Check sheet for the modelled part. Datum: model origin and axes. Units: mm. A direction names the side the tool comes from. Give positions to 0.01 mm unless a question says otherwise; leave off trailing zeros. Order: outer loops, then holes, each group sorted by start corner. A loop starts at its lowest first (then second) coordinate and runs counter-clockwise, first axis right, second up. Notation, with made-up numbers: (-25.5, 15) - (-0.5, 15) arc R25 ccw to (-0.5, 30) - close; hole circle Ø10 at (-28.5, 14.5). An arc over 180 degrees is marked (long way). Answer in a Markdown table with one row per item.
from build123d import *

# Parameters (mm, degrees)
F0_W     = 527.05
F0_H     = 190.5
F1_DEPTH = 38.1
F3_DEPTH = 12.7


# Not quite as in the source:
# - a pattern or mirror of a feature is missing from the dataset's text; its kind, count and spacing are read off the source's solid


with BuildPart() as f1:
    # F0 (on Top) → F1 (new body, symmetric)
    with BuildSketch(Plane.XY):
        Rectangle(F0_W, F0_H)
    extrude(amount=F1_DEPTH, both=True)

    # F2 (on face) → F3 (cut)
    with BuildSketch(Plane(origin=(0, 0, -38.1), x_dir=(1, 0, 0), z_dir=(0, 0, -1))):
        Polygon((250.825, 95.25), (-250.825, 95.25), (-250.825, 82.55), (-263.525, 82.55), (-263.525, -82.55), (-250.825, -82.55), (-250.825, -95.25), (250.825, -95.25), (250.825, -82.55), (263.525, -82.55), (263.525, 82.55), (250.825, 82.55), align=None)
    f3 = extrude(amount=-F3_DEPTH, mode=Mode.SUBTRACT)

    # F3_copies: F3 across plane
    add(f3.mirror(Plane.XY), mode=Mode.SUBTRACT)


solid = f1.part
(1) Access from +Z, -Z, +X, -X, +Y, -Y to the whole of each face (thin tool, end or side, straight path). Record for faces 1 (the flat face through (-250.825, 89, -32)), 2 (the flat face through (-257, 82.55, -32)), 3 (the flat face through (-257, -82.55, 32)).
Geometry says:
| item | result |
|---|---|
| face 1 | -Z, +Y, -Y |
| face 2 | -Z, +X, -X |
| face 3 | +Z, +X, -X |
(2) Gauge pin test, flat ends, axial feed: P1, Ø4, axis at x = -57, y = -50, coming from the -Z side; P2, Ø6, axis at x = -1.5, y = -25, coming from the +Z side. Record the tip position at first contact, or that the pin passes through.
Geometry says:
| item | result |
|---|---|
| P1 | z = -25.4 |
| P2 | z = 25.4 |
(3) Cross-section at A-A, the plane z = -30.5. Record the cut outline in (x, y) (3 decimals), then the cut area to 3 significant figures.
Geometry says:
| item | result |
|---|---|
| outline | (-263.525, -95.25) - (-250.825, -95.25) - (-250.825, -82.55) - (-263.525, -82.55) - close; (-263.525, 82.55) - (-250.825, 82.55) - (-250.825, 95.25) - (-263.525, 95.25) - close; (250.825, -95.25) - (263.525, -95.25) - (263.525, -82.55) - (250.825, -82.55) - close; (250.825, 82.55) - (263.525, 82.55) - (263.525, 95.25) - (250.825, 95.25) - close |
| area | 645 mm² |
(4) Mould release check, pull along Y, two halves, no side actions. Record for faces 4 (the flat face through (-250.825, -89, 32)), 5 (the flat face through (257, 82.55, -32)): pulls with the +Y half, pulls with the -Y half, needs draft (parallel to the pull), parting line crosses it, or undercut.
Geometry says:
| item | result |
|---|---|
| face 4 | needs draft |
| face 5 | undercut |
(5) Thickness scan on L1, parallel to X at y = 87.5, z = -28.5 (3 decimals); L2, parallel to Z at x = 107.5, y = 24.5. Record the ranges inside material, lowest first.
Geometry says:
| item | result |
|---|---|
| L1 | -263.525 to -250.825, 250.825 to 263.525 |
| L2 | -25.4 to 25.4 |
(6) Cross-section at B-B, the plane x = -101.5. Record the cut outline in (y, z).
Geometry says:
| item | result |
|---|---|
| outline | (-95.25, -25.4) - (95.25, -25.4) - (95.25, 25.4) - (-95.25, 25.4) - close |
(7) Cross-section at C-C, the plane y = 36. Record the cut outline in (x, z) (3 decimals).
Geometry says:
| item | result |
|---|---|
| outline | (-263.525, -25.4) - (263.525, -25.4) - (263.525, 25.4) - (-263.525, 25.4) - close |
